The model under review builds one solid part; all positions refer to its coordinate system, in mm. Give positions to 0.01 mm unless a question says otherwise; leave off trailing zeros. Write each loop counter-clockwise with the first axis right and the second up, starting at its lowest first coordinate (ties: lowest second). Pieces come first, ordered by that corner, then holes. Notation, with made-up numbers: (76, -39) - (97, -39) arc R25 ccw to (97, -26) - close; hole circle Ø3 at (70.5, -1.75). An arc over 180 degrees is marked (long way). One line per question, with ' | ' between items. Start each with the question number.
```python
from build123d import *

# Parameters (mm, degrees)
BOSS_EXTRUDE1_DEPTH = 1.499997834
BOSS_EXTRUDE2_DEPTH = 2.999998821
CUT_EXTRUDE1_DEPTH  = 2.999999995
FILLET1_R           = 1.400201404
BOSS_EXTRUDE3_REACH = 8499.621
SKETCH4_W           = 6.8
SKETCH4_H           = 1


with BuildPart() as part:
    # Sketch1 → Boss-Extrude1 (new body)
    with BuildSketch(Plane(origin=(-3679.783466787, -3e-09, -4864.000529017), x_dir=(0, -1, 0), z_dir=(-0.6033298825291362, -4.862971078225009e-13, -0.7974917258801991))):
        with BuildLine():
            Line((-531.630972559, 8466.305810109), (-709.630972559, 8466.305810109))
            ThreePointArc((-709.630972559, 8466.305810109), (-713.873613004, 8464.548451039), (-715.630972559, 8460.305810795))
            ThreePointArc((-715.630972559, 8460.305810795), (-713.873613489, 8456.063169664), (-709.630972559, 8454.305810109))
            Line((-709.630972559, 8454.305810109), (-531.630972559, 8454.305810109))
            ThreePointArc((-531.630972559, 8454.305810109), (-525.630972559, 8460.305810109), (-531.630972559, 8466.305810109))
        make_face()
    extrude(amount=-BOSS_EXTRUDE1_DEPTH)

    # Sketch2 → Boss-Extrude2 (add)
    with BuildSketch(Plane(origin=(-3679.783466787, -3e-09, -4864.000529017), x_dir=(-0.7974917258801992, 3.679004651903849e-13, 0.6033298825291362), z_dir=(-0.6033298825291362, -4.862971078225007e-13, -0.7974917258801992))):
        with BuildLine():
            Line((8455.40581011, 531.630972551), (8455.40581011, 709.630972551))
            ThreePointArc((8455.40581011, 709.630972551), (8456.840986746, 713.095795642), (8460.305809725, 714.530972551))
            ThreePointArc((8460.305809725, 714.530972551), (8463.770633201, 713.095795914), (8465.20581011, 709.630972551))
            Line((8465.20581011, 709.630972551), (8465.20581011, 531.630972551))
            ThreePointArc((8465.20581011, 531.630972551), (8460.30581011, 526.730972551), (8455.40581011, 531.630972551))
        make_face()
    extrude(amount=BOSS_EXTRUDE2_DEPTH)

    # Sketch3 → Cut-Extrude1 (cut)
    with BuildSketch(Plane(origin=(-3681.593455723, -3e-09, -4866.393003255), x_dir=(-0.7974917258801991, 3.6790046519038474e-13, 0.6033298825291363), z_dir=(-0.6033298825291363, -4.862971078225009e-13, -0.7974917258801992))):
        with BuildLine():
            Line((8463.705809388, 531.630972551), (8463.705809388, 709.630972551))
            ThreePointArc((8463.705809388, 709.630972551), (8462.709972444, 712.035135607), (8460.305809388, 713.030972551))
            ThreePointArc((8460.305809388, 713.030972551), (8457.901646332, 712.035135607), (8456.905809388, 709.630972551))
            Line((8456.905809388, 709.630972551), (8456.905809388, 531.630972551))
            ThreePointArc((8456.905809388, 531.630972551), (8460.305809388, 528.230972551), (8463.705809388, 531.630972551))
        make_face()
    extrude(amount=-CUT_EXTRUDE1_DEPTH, mode=Mode.SUBTRACT)

    # Fillet1
    fillet1_edges = [part.edges().sort_by_distance(p)[0] for p in [
        (-10422.518884598, 713.87361348, 238.991305657),
        (-10421.117404893, 620.630972551, 237.931038123),
        (-10425.902355248, 525.630972551, 241.551017418),
        (-10430.687305604, 620.630972551, 245.170996713),
    ]]
    fillet(fillet1_edges, radius=FILLET1_R)

    # Sketch4 → Boss-Extrude3 (add, up to next)
    with BuildSketch(Plane(origin=(-3681.593455723, -3e-09, -4866.393003255), x_dir=(-0.7974917258801991, 3.679004651903847e-13, 0.6033298825291363), z_dir=(-0.6033298825291363, -4.862971078225008e-13, -0.7974917258801992)), mode=Mode.PRIVATE) as boss_extrude3_sk1:
        with Locations((8460.305809388, 682.230972551)):
            Rectangle(SKETCH4_W, SKETCH4_H)
    boss_extrude3_tool1 = extrude(boss_extrude3_sk1.sketch, amount=-BOSS_EXTRUDE3_REACH, mode=Mode.PRIVATE) - part.part
    # Sketch4 → Boss-Extrude3 (add, up to next)
    with BuildSketch(Plane(origin=(-3681.593455723, -3e-09, -4866.393003255), x_dir=(-0.7974917258801991, 3.679004651903847e-13, 0.6033298825291363), z_dir=(-0.6033298825291363, -4.862971078225008e-13, -0.7974917258801992)), mode=Mode.PRIVATE) as boss_extrude3_sk2:
        with Locations((8460.305809388, 651.430972551)):
            Rectangle(SKETCH4_W, SKETCH4_H)
    boss_extrude3_tool2 = extrude(boss_extrude3_sk2.sketch, amount=-BOSS_EXTRUDE3_REACH, mode=Mode.PRIVATE) - part.part
    # Sketch4 → Boss-Extrude3 (add, up to next)
    with BuildSketch(Plane(origin=(-3681.593455723, -3e-09, -4866.393003255), x_dir=(-0.7974917258801991, 3.679004651903847e-13, 0.6033298825291363), z_dir=(-0.6033298825291363, -4.862971078225008e-13, -0.7974917258801992)), mode=Mode.PRIVATE) as boss_extrude3_sk3:
        with Locations((8460.305809388, 620.630972551)):
            Rectangle(SKETCH4_W, SKETCH4_H)
    boss_extrude3_tool3 = extrude(boss_extrude3_sk3.sketch, amount=-BOSS_EXTRUDE3_REACH, mode=Mode.PRIVATE) - part.part
    # Sketch4 → Boss-Extrude3 (add, up to next)
    with BuildSketch(Plane(origin=(-3681.593455723, -3e-09, -4866.393003255), x_dir=(-0.7974917258801991, 3.679004651903847e-13, 0.6033298825291363), z_dir=(-0.6033298825291363, -4.862971078225008e-13, -0.7974917258801992)), mode=Mode.PRIVATE) as boss_extrude3_sk4:
        with Locations((8460.305809388, 589.830972551)):
            Rectangle(SKETCH4_W, SKETCH4_H)
    boss_extrude3_tool4 = extrude(boss_extrude3_sk4.sketch, amount=-BOSS_EXTRUDE3_REACH, mode=Mode.PRIVATE) - part.part
    # Sketch4 → Boss-Extrude3 (add, up to next)
    with BuildSketch(Plane(origin=(-3681.593455723, -3e-09, -4866.393003255), x_dir=(-0.7974917258801991, 3.679004651903847e-13, 0.6033298825291363), z_dir=(-0.6033298825291363, -4.862971078225008e-13, -0.7974917258801992)), mode=Mode.PRIVATE) as boss_extrude3_sk5:
        with Locations((8460.305809388, 559.030972551)):
            Rectangle(SKETCH4_W, SKETCH4_H)
    boss_extrude3_tool5 = extrude(boss_extrude3_sk5.sketch, amount=-BOSS_EXTRUDE3_REACH, mode=Mode.PRIVATE) - part.part
    add(boss_extrude3_tool1.solids().sort_by_distance((-10428.617337, 682.230973, 237.962307))[0])
    add(boss_extrude3_tool2.solids().sort_by_distance((-10428.617337, 651.430973, 237.962307))[0])
    add(boss_extrude3_tool3.solids().sort_by_distance((-10428.617337, 620.630973, 237.962307))[0])
    add(boss_extrude3_tool4.solids().sort_by_distance((-10428.617337, 589.830973, 237.962307))[0])
    add(boss_extrude3_tool5.solids().sort_by_distance((-10428.617337, 559.030973, 237.962307))[0])


solid = part.part
```
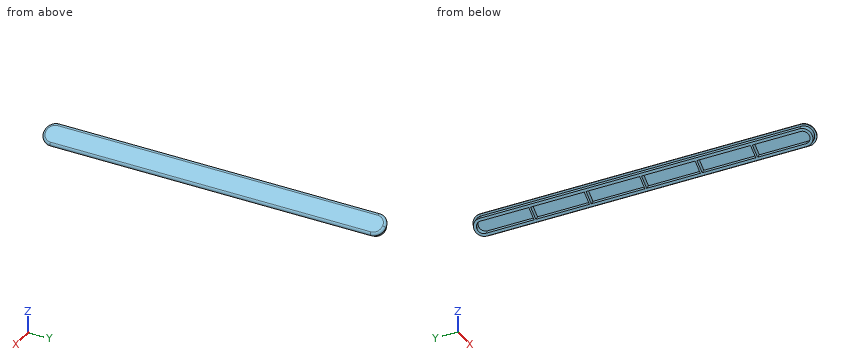
Item 1: Take a section at A-A (y = 704). Give the boundary of the cut face in (x, z).
Item 2: For probe 1 along X at (y, z) = (664, 241); probe 2 along X at (y, z) = (609.5, 240.25); probe 3 along Z at (x, y) = (-10425.75, 591), list the stretches that pass through material, from the lowest coordinate up.
Item 3: Clearance check with flat-ended pins moving along their axes: P1, Ø3, axis at x = -10429, z = 239.5, coming from the -Y side; P2, Ø3, axis at x = -10429, z = 240.5, coming from the -Y side; P3, Ø1.5, axis at y = 628, z = 240, coming from the -X side. State where each tip first meets the part, or that it passes through.
Check sheet entries:
1) outline: (-10432.53, 240.92) - (-10431.33, 240.01) - (-10429.52, 242.41) - (-10424.1, 238.3) - (-10425.91, 235.91) - (-10424.71, 235.01) - (-10422.9, 237.4) - (-10422.02, 236.73) - (-10421.96, 236.81) arc R1.4 ccw to (-10422.23, 238.78) - (-10429.57, 244.33) arc R1.4 ccw to (-10431.53, 244.05) - (-10431.59, 243.97) - (-10430.72, 243.31) - close
2) probe 1: x = -10432.46 to -10430.58, -10427.66 to -10425.17 | probe 2: x = -10431.64 to -10431.15, -10426.67 to -10424.18 | probe 3: z = 235.79 to 236.12, 239.55 to 241.44
3) P1: stops at y = 526.73 | P2: stops at y = 525.71 | P3: stops at x = -10432.3
